Build history of the part. All positions in model axes, mm. Face numbers are marked on the shaded views. A direction names the side the tool comes from. Coordinates: 2 decimals unless noted, no trailing zeros. Loops run counter-clockwise (first coordinate to the right, second up) from the corner with the lowest first, then second, coordinate; pieces in that order, holes last.
Item 1: Cut at A-A (z = 12.25). List the corners of the cut face in (x, y), and give its area (3 significant figures).
Item 2: Mould opens along Y. For the marked faces 3, 4 and 5 say: released by +Y, released by -Y, zero draft, split by the parting line, or undercut.
Item 3: 3-axis set-ups, long thin cutter, end or side, ignore diameter. For the marked faces 1 and 2: which of +Z, -Z, +X, -X, +Y, -Y reach the whole face in a straight line?
Item 4: Drill centre lines: line 1 along Y through (x, z) = (-18, 13.75); line 2 along X through (y, z) = (-8.5, 6.5); line 3 along Z through (x, y) = (-11.5, 4.75). Where is each one in solid material? Low to high.
Item 5: Cut at C-C (y = 0). List the corners of the cut face in (x, z).
Item 6: Flat gauge pins, fed straight in: pin 1 (6 mm diameter, centred on x = 8, y = 0.5, fed in from +Z); pin 2 (1.1 mm diameter, centred on x = -29.5, z = 14, fed in from -Y); pin 3 (1.1 mm diameter, centred on x = -0.5, y = -3.5, fed in from +Z). Where does each tip first touch, or does it go through?
Item 7: Cut at D-D (z = 7.75). List the corners of the cut face in (x, y), and give its area (3 significant figures).
Item 8: Cut at B-B (x = 14). List the corners of the cut face in (y, z).
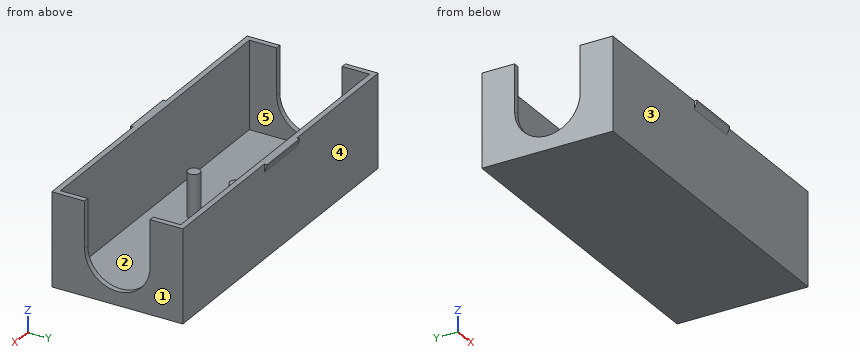
from build123d import *

# Parameters (mm, degrees)
F0_W      = 60
F0_H      = 24
F1_DEPTH  = 17
F2_T      = -1
F3_W      = 10
F3_H      = 1.5
F4_DEPTH  = 0.5
F5_SIZE2  = 1.19999
F5_SIZE   = 0.49999
F8_DEPTH  = 60.001
F9_R      = 1.1
F10_DEPTH = 8


# Not quite as in the source:
# - a fillet or chamfer is up to 0.001 mm smaller than in the source, because OpenCascade refuses the exact size


with BuildPart() as f1:
    # F0 (on Top) → F1 (new body)
    with BuildSketch(Plane.XY):
        Rectangle(F0_W, F0_H)
    extrude(amount=F1_DEPTH)

    # F2
    f2_openings = [f1.faces().sort_by_distance(p)[0] for p in [
        (0, 0, 17),
    ]]
    offset(amount=F2_T, openings=f2_openings)

    # F3 (on face) → F4 (join)
    with BuildSketch(Plane.XZ.offset(12)):
        with Locations((0, 16.25)):
            Rectangle(F3_W, F3_H)
    extrude(amount=F4_DEPTH)

    # F5 (size 0.5 and 1.2 in the source; OpenCascade refuses exactly that, so slightly less here)
    f5_edges = [f1.edges().sort_by_distance(p)[0] for p in [
        (0, -12.5, 15.5),
    ]]
    f5_side = f1.faces().sort_by_distance((0, -12.25, 15.5))[0]
    chamfer(f5_edges, length=F5_SIZE, length2=F5_SIZE2, reference=f5_side)

    # F6: F1 across plane


with BuildPart() as f1_1:
    add(f1.part)
    add(f1.part.mirror(Plane.XZ))

    # F7 (on face) → F8 (cut, through all)
    with BuildSketch(Plane(origin=(-30, 0, 0), x_dir=(0, -1, 0), z_dir=(-1, 0, 0))):
        with BuildLine():
            Line((-6, 17), (-6, 8.5))
            ThreePointArc((-6, 8.5), (0, 2.5), (6, 8.5))
            Line((6, 8.5), (6, 17))
            Line((6, 17), (-6, 17))
        make_face()
    extrude(amount=-F8_DEPTH, mode=Mode.SUBTRACT)

    # F9 (on face) → F10 (join)
    with BuildSketch(Plane.XY.offset(1)):
        with Locations((0, 3.85)):
            Circle(F9_R)
        with Locations((0, -3.85)):
            Circle(F9_R)
    extrude(amount=F10_DEPTH)


solid = f1_1.part
Filled sheet:
1. outline: (-30, -12) - (30, -12) - (30, -6) - (29, -6) - (29, -11) - (-29, -11) - (-29, -6) - (-30, -6) - close; (-30, 6) - (-29, 6) - (-29, 11) - (29, 11) - (29, 6) - (30, 6) - (30, 12) - (-30, 12) - close
1. area: 140 mm2
2. face 3: released by -Y
2. face 4: released by +Y
2. face 5: undercut
3. face 1: +Z, -Z, +X, +Y, -Y
3. face 2: +Z
4. line 1: y = -12 to -11, 11 to 12
4. line 2: x = -30 to -29, 29 to 30
4. line 3: z = 0 to 1
5. outline: (-30, 0) - (30, 0) - (30, 2.5) - (29, 2.5) - (29, 1) - (-29, 1) - (-29, 2.5) - (-30, 2.5) - close
6. pin 1: stops at z = 1
6. pin 2: stops at y = -12
6. pin 3: stops at z = 9
7. outline: (-30, -12) - (30, -12) - (30, -5.95) - (29, -5.95) - (29, -11) - (-29, -11) - (-29, -5.95) - (-30, -5.95) - close; (-30, 5.95) - (-29, 5.95) - (-29, 11) - (29, 11) - (29, 5.95) - (30, 5.95) - (30, 12) - (-30, 12) - close; circle Ø2.2 at (0, -3.85); circle Ø2.2 at (0, 3.85)
7. area: 148 mm2
8. outline: (-12, 0) - (12, 0) - (12, 17) - (11, 17) - (11, 1) - (-11, 1) - (-11, 17) - (-12, 17) - close
